Part model, mm, in its own coordinate system. Face numbers are marked on the shaded views. A direction names the side the tool comes from. Round coordinates to 2 decimals unless told otherwise and drop trailing zeros. Loops run counter-clockwise (first coordinate to the right, second up) from the corner with the lowest first, then second, coordinate; pieces in that order, holes last. Notation, with made-up numbers: (-16.5, 26) - (29.5, 26) arc R32 ccw to (29.5, 62) - close; hole circle Ø11 at (21, -12.75). An arc over 180 degrees is marked (long way). Put each result on its own line as item: value.
Solid Edge part; units mm, degrees
sketch "Sketch1" plane through (0, 0, 0) normal (0, -1, 0) x (1, 0, 0)
  line L0 (-175, -5) -> (175, -5)
  line L1 (175, -5) -> (175, 5)
  line L2 (175, 5) -> (-175, 5)
  line L3 (-175, 5) -> (-175, -5)
  dimension "D1" = 175
  dimension "D2" = 175
extrude "Protrusion1" add sketch "Sketch1" against normal blind 200
sketch "Sketch2" plane through (0, 100, -5) normal (0, 0, -1) x (1, 0, 0)
  line L0 (-22.8, 78.97) -> (-22.8, 72.97)
  line L1 (-22.8, 72.97) -> (-18.3, 72.97)
  line L2 (-18.3, 72.97) -> (-18.3, 78.97)
  line L3 (-18.3, 78.97) -> (-15.3, 78.97)
  line L4 (-15.3, 78.97) -> (-10.3, 78.97)
  line L5 (-10.3, 78.97) -> (-10.3, 93.97)
  line L6 (-10.3, 93.97) -> (-15.3, 93.97)
  line L7 (-15.3, 93.97) -> (-15.3, 101.97)
  line L8 (-15.3, 101.97) -> (-18.3, 101.97)
  line L9 (-18.3, 101.97) -> (-18.3, 107.97)
  line L10 (-18.3, 107.97) -> (-22.8, 107.97)
  line L11 (-22.8, 107.97) -> (-22.8, 101.97)
  line L12 (-22.8, 101.97) -> (-37.8, 101.97)
  line L13 (-37.8, 101.97) -> (-37.8, 78.97)
  line L14 (-37.8, 78.97) -> (-35.3, 78.97)
  line L15 (-35.3, 78.97) -> (-35.3, 70.97)
  line L16 (-35.3, 70.97) -> (-30.3, 70.97)
  line L17 (-30.3, 70.97) -> (-30.3, 78.97)
  line L18 (-30.3, 78.97) -> (-22.8, 78.97)
  dimension "D1" = 37.8
  dimension "D2" = 22.8
  dimension "D3" = 18.3
  dimension "D4" = 15.3
  dimension "D5" = 10.3
  dimension "D6" = 35.3
  dimension "D7" = 35.3
extrude "Cutout1" cut sketch "Sketch2" against normal blind 8
sketch "Sketch3" plane through (0, 100, -5) normal (0, 0, -1) x (1, 0, 0)
  line L0 (11, 72.97) -> (-11, 72.97)
  line L1 (-11, 111.97) -> (-11, 72.97)
  line L2 (11, 111.97) -> (-11, 111.97)
  line L3 (11, 111.97) -> (11, 72.97)
  dimension "D1" = 11
  dimension "D2" = 11
extrude "Cutout2" cut sketch "Sketch3" against normal through all
mirror "Mirror1" about plane through (0, 100, 0) normal (0, -1, 0) of "Cutout1", "Cutout2"
mirror "Mirror2" about plane through (40, 0, 0) normal (1, 0, 0) of "Mirror1", "Cutout2", "Cutout1"
mirror "Mirror3" about plane through (-40, 0, 0) normal (1, 0, 0) of "Cutout2", "Cutout1", "Mirror1"
sketch "Sketch4" plane through (0, 100, -5) normal (0, 0, -1) x (0, -1, 0)
  line L0 (-22.6, 109.45) -> (-22.6, 103.45)
  line L1 (-22.6, 103.45) -> (-18.1, 103.45)
  line L2 (-18.1, 103.45) -> (-18.1, 109.45)
  line L3 (-18.1, 109.45) -> (-15.1, 109.45)
  line L4 (-15.1, 109.45) -> (-11, 109.45)
  line L5 (-11, 109.45) -> (-11, 124.45)
  line L6 (-11, 124.45) -> (-15.1, 124.45)
  line L7 (-15.1, 124.45) -> (-15.1, 131.95)
  line L8 (-15.1, 131.95) -> (-18.1, 131.95)
  line L9 (-18.1, 131.95) -> (-18.1, 137.95)
  line L10 (-18.1, 137.95) -> (-22.6, 137.95)
  line L11 (-22.6, 137.95) -> (-22.6, 131.95)
  line L12 (-22.6, 131.95) -> (-37.6, 131.95)
  line L13 (-37.6, 131.95) -> (-37.6, 109.45)
  line L14 (-37.6, 109.45) -> (-35.1, 109.45)
  line L15 (-35.1, 109.45) -> (-35.1, 101.45)
  line L16 (-35.1, 101.45) -> (-30.1, 101.45)
  line L17 (-30.1, 101.45) -> (-30.1, 109.45)
  line L18 (-30.1, 109.45) -> (-22.6, 109.45)
  dimension "D1" = 22.6
  dimension "D2" = 18.1
  dimension "D3" = 15.1
  dimension "D4" = 11
  dimension "D5" = 37.6
  dimension "D6" = 35.1
  dimension "D7" = 35.1
  dimension "D8" = 37.6
  dimension "D9" = 22.6
extrude "Cutout3" cut sketch "Sketch4" against normal up to vertex (8 mm away)
sketch "Sketch5" plane through (0, 100, -5) normal (0, 0, -1) x (0, -1, 0)
  line L0 (-11, 109.45) -> (-11, 103.45)
  line L1 (-11, 103.45) -> (11, 103.45)
  line L2 (11, 103.45) -> (11, 175)
  line L3 (11, 175) -> (-11, 175)
  line L4 (-11, 175) -> (-11, 109.45)
  dimension "D1" = 11
  dimension "D2" = 11
extrude "Cutout4" cut sketch "Sketch5" against normal through all
mirror "Mirror4" about plane through (0, 0, 0) normal (1, 0, 0) of "Cutout4", "Cutout3"
sketch "Sketch6" plane through (0, 100, -5) normal (0, 0, -1) x (1, 0, 0)
  circle A0 centre (-97.5, 62.5) radius 1.875
  circle A1 centre (-52.5, 62.5) radius 1.875
  circle A2 centre (-52.5, 0) radius 1.875
  circle A3 centre (-97.5, -62.5) radius 1.875
  circle A4 centre (-52.5, -62.5) radius 1.875
  dimension "D1" = 97.5
  dimension "D2" = 97.5
extrude "Cutout5" cut sketch "Sketch6" against normal blind 7
sketch "Sketch7" plane through (0, 100, 5) normal (0, 0, 1) x (1, 0, 0)
  line L0 (-120, 84) -> (-120, 44)
  line L1 (-120, 44) -> (-145, 44)
  line L2 (-145, 44) -> (-145, 84)
  line L3 (-145, 84) -> (-120, 84)
  dimension "D1" = 145
  dimension "D2" = 145
extrude "Cutout6" cut sketch "Sketch7" against normal blind 5
mirror "Mirror5" about plane through (0, 100, 0) normal (0, -1, 0) of "Cutout6"
mirror "Mirror6" about plane through (0, 0, 0) normal (1, 0, 0) of "Cutout6", "Mirror5"
sketch "Sketch8" plane through (0, 100, 5) normal (0, 0, 1) x (1, 0, 0)
  line L0 (21, 100) -> (21, -100)
extrude "Cutout7" cut sketch "Sketch8" against normal through all material side at (20.95, 100, 5)
properties material "Nylon, allgemein"
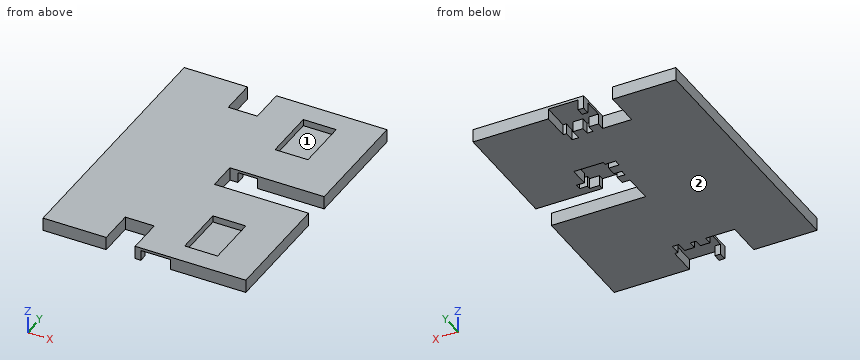
1. Band-saw the part on B-B (x = 159). List the corners of the cut face in (y, z).
A:
outline: (0, -5) - (89, -5) - (89, 5) - (0, 5) - close; (111, -5) - (200, -5) - (200, 5) - (111, 5) - close
2. Band-saw the part on A-A (y = 13). List the corners of the cut face in (x, z), plus the area to 3 significant figures.
A:
outline: (21, -5) - (69, -5) - (69, 5) - (21, 5) - close; (91, 3) - (117.8, 3) - (117.8, -5) - (175, -5) - (175, 5) - (91, 5) - close
area: 1,110 mm²
3. Band-saw the part on D-D (z = -2). Give the number of separate pieces and of enclosed holes in the cut face, plus the area to 3 significant figures.
A:
separate pieces: 3
enclosed holes: 0
area: 26,200 mm²
4. Tool access for the marked faces 1 and 2: list every direction of +Z, -Z, +X, -X, +Y, -Y with a clear straight run to the whole face (end or side of a thin tool).
A:
face 1: +Z
face 2: -Z, +X, -X, +Y, -Y
5. Probe line 1 along Y through (x, z) = (93.5, -3.75); line 2 along Y through (x, z) = (138.5, 2.5); line 3 along X through (y, z) = (24, -2.25). List the from-to ranges inside material, lowest first. Write a range as [from, to].
A:
line 1: y = [0, 6.03], [21.03, 178.97], [193.97, 200]
line 2: y = [0, 16], [56, 89], [111, 144], [184, 200]
line 3: x = [21, 69], [91, 98.3], [102.8, 110.3], [115.3, 175]
6. Band-saw the part on C-C (y = 126.5). List the corners of the cut face in (x, z).
A:
outline: (21, -5) - (109.45, -5) - (109.45, 3) - (131.95, 3) - (131.95, -5) - (175, -5) - (175, 5) - (21, 5) - close
7. Pin check, flat tips, straight feed: P1, Ø5, axis at x = 100.5, z = -1, coming from the +Y side; P2, Ø1.2, axis at x = 116.5, z = 0, coming from the -Y side. Stop position of each tip, or through.
A:
P1: stops at y = 178.97
P2: stops at y = 21.03
